Geometry check sheet. Reference: the model listing, model coordinates, mm. Face numbers are marked on the shaded views. Give positions to 0.01 mm unless a question says otherwise; leave off trailing zeros. Write each loop counter-clockwise with the first axis right and the second up, starting at its lowest first coordinate (ties: lowest second). Pieces come first, ordered by that corner, then holes.
(1) Depth check by flat-ended pin: P1, Ø7, axis at x = 26.5, z = 36.5, coming from the -Y side. Enter the tip coordinate at first touch or a pass-through.
(2) Mould release check, pull along Z, two halves, no side actions. Record for the marked faces 1, 2 and 3: +Z half, -Z half, draft (parallel to the pull), parting line (faces both ways), or undercut.
(3) Cross-section at B-B (y = -46). Record the boundary of the cut face in (x, z) (3 decimals).
(4) Cross-section at D-D (x = 24.5). Record the boundary of the cut face in (y, z).
(5) Thickness scan on line 1 along X through (y, z) = (-2, -39.5); line 2 along X through (y, z) = (-21, -35); line 3 along Z through (x, y) = (23, -43) (3 decimals). Record the ranges inside material, lowest first.
(6) Cross-section at A-A (z = 0). Record the boundary of the cut face in (x, y), and give its area (3 significant figures).
(7) Cross-section at C-C (x = 9.5). Record the boundary of the cut face in (y, z) (3 decimals), and give its area (3 significant figures).
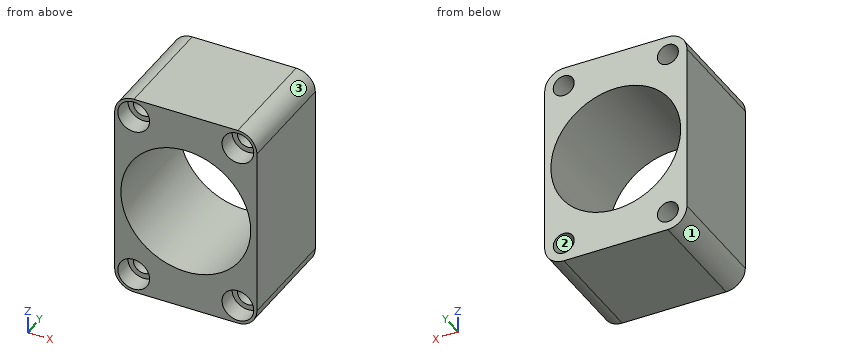
```python
from build123d import *

# Parameters (mm, degrees)
F0_W     = 63.86
F0_H     = 92.75
F1_DEPTH = 49.45
F2_R     = 8.6
F3_R     = 4.705062
F4_DEPTH = 54.1
F5_R     = 7.125
F6_DEPTH = 8.5
F7_R     = 29.15
F8_DEPTH = 69.1


with BuildPart() as f1:
    # F0 (on Front) → F1 (new body)
    with BuildSketch(Plane.XZ):
        Rectangle(F0_W, F0_H)
    extrude(amount=F1_DEPTH)

    # F2
    f2_edges = [f1.edges().sort_by_distance(p)[0] for p in [
        (31.93, -24.725, 46.375),
        (-31.93, -24.725, 46.375),
        (-31.93, -24.725, -46.375),
        (31.93, -24.725, -46.375),
    ]]
    fillet(f2_edges, radius=F2_R)

    # F3 (on face) → F4 (cut)
    with BuildSketch(Plane.XZ.offset(49.45)):
        with Locations((-23.4, 37.9)):
            Circle(F3_R)
        with Locations((23.4, 37.9)):
            Circle(F3_R)
        with Locations((-23.4, -37.9)):
            Circle(F3_R)
        with Locations((23.4, -37.9)):
            Circle(F3_R)
    extrude(amount=-F4_DEPTH, mode=Mode.SUBTRACT)

    # F5 (on face) → F6 (cut)
    with BuildSketch(Plane.XZ.offset(49.45)):
        with Locations((-23.4, 37.9)):
            Circle(F5_R)
        with Locations((23.4, 37.9)):
            Circle(F5_R)
        with Locations((-23.4, -37.9)):
            Circle(F5_R)
        with Locations((23.4, -37.9)):
            Circle(F5_R)
    extrude(amount=-F6_DEPTH, mode=Mode.SUBTRACT)

    # F7 (on face) → F8 (cut)
    with BuildSketch(Plane.XZ.offset(49.45)):
        Circle(F7_R)
    extrude(amount=-F8_DEPTH, mode=Mode.SUBTRACT)


solid = f1.part
```
Reply:
1. P1: stops at y = -40.95
2. face 1: -Z half
2. face 2: undercut
2. face 3: +Z half
3. outline: (-31.93, -37.775) arc R8.6 ccw to (-23.33, -46.375) - (23.33, -46.375) arc R8.6 ccw to (31.93, -37.775) - (31.93, 37.775) arc R8.6 ccw to (23.33, 46.375) - (-23.33, 46.375) arc R8.6 ccw to (-31.93, 37.775) - close; hole circle Ø14.25 at (-23.4, -37.9); hole circle Ø14.25 at (-23.4, 37.9); hole circle Ø58.3 at (0, 0); hole circle Ø14.25 at (23.4, -37.9); hole circle Ø14.25 at (23.4, 37.9)
4. outline: (-49.45, -46.3) - (0, -46.3) - (0, -42.47) - (-40.95, -42.47) - (-40.95, -44.94) - (-49.45, -44.94) - close; (-49.45, -30.86) - (-40.95, -30.86) - (-40.95, -33.33) - (0, -33.33) - (0, -15.79) - (-49.45, -15.79) - close; (-49.45, 15.79) - (0, 15.79) - (0, 33.33) - (-40.95, 33.33) - (-40.95, 30.86) - (-49.45, 30.86) - close; (-49.45, 44.94) - (-40.95, 44.94) - (-40.95, 42.47) - (0, 42.47) - (0, 46.3) - (-49.45, 46.3) - close
5. line 1: x = -31.76 to -27.82, -18.98 to 18.98, 27.82 to 31.76
5. line 2: x = -31.93 to -27.11, -19.69 to 19.69, 27.11 to 31.93
5. line 3: z = -46.375 to -45.014, -30.786 to -17.909, 17.909 to 30.786, 45.014 to 46.375
6. outline: (-31.93, -49.45) - (-29.15, -49.45) - (-29.15, 0) - (-31.93, 0) - close; (29.15, -49.45) - (31.93, -49.45) - (31.93, 0) - (29.15, 0) - close
6. area: 275 mm2
7. outline: (-49.45, -46.375) - (0, -46.375) - (0, -27.559) - (-49.45, -27.559) - close; (-49.45, 27.559) - (0, 27.559) - (0, 46.375) - (-49.45, 46.375) - close
7. area: 1,860 mm2
